The listing builds one solid part. Answer for the finished solid, in the listing's coordinates (mm). Round coordinates to 2 decimals unless told otherwise and drop trailing zeros. Write each loop counter-clockwise with the first axis right and the second up, starting at its lowest first coordinate (ties: lowest second). Pieces come first, ordered by that corner, then holes. Notation, with made-up numbers: (31, 47) - (77, 47) arc R26 ccw to (77, 71) - close; hole circle Ø4 at (69.5, -20.5). An arc over 180 degrees is marked (long way). Answer in a Markdown table with one row per item.
Autodesk Inventor part; units mm, degrees
ref_plane "YZ Plane" through (0, 0, 0) normal (1, 0, 0) x (0, 1, 0)
ref_plane "XZ Plane" through (0, 0, 0) normal (0, 1, 0) x (-1, 0, 0)
ref_plane "XY Plane" through (0, 0, 0) normal (0, 0, 1) x (1, 0, 0)
sketch "board" plane through (0, 0, 0) normal (0, 0, 1) x (1, 0, 0)
  line L0 (22.5, 10) -> (-22.5, 10)
  line L1 (-22.5, 10) -> (-22.5, -10)
  line L2 (-22.5, -10) -> (22.5, -10)
  line L3 (22.5, -10) -> (22.5, 10)
  line L4 (22.5, 10) -> (-22.5, -10) construction
  line L5 (-22.5, 10) -> (22.5, -10) construction
  circle A0 centre (-3.81, -8) radius 0.5
  circle A1 centre (-21.25, 8.75) radius 0.8
  circle A2 centre (21.25, 8.75) radius 0.8
  circle A3 centre (-21.25, -8.75) radius 0.8
  circle A4 centre (21.25, -8.75) radius 0.8
  circle A5 centre (-1.27, -8) radius 0.5
  circle A6 centre (1.27, -8) radius 0.5
  circle A7 centre (3.81, -8) radius 0.5
  circle A8 centre (-2.44, 7) radius 0.5
  circle A9 centre (2.44, 7) radius 0.5
  circle A10 centre (-13.1, 5.1) radius 0.75
  circle A11 centre (13.1, 5.1) radius 0.75
  circle A12 centre (-13.1, -5.1) radius 0.75
  circle A13 centre (13.1, -5.1) radius 0.75
  point P0 (0, 0)
  point P1 (0, 0)
  point P2 (13.2529, 5)
  dimension "d34" = 45
  dimension "d35" = 20
  dimension "d39" = 1
  dimension "d44" = 1.6
  dimension "d48" = 1.25
  dimension "d51" = 42.5
  dimension "d54" = 17.5
  dimension "d57" = 1.25
  dimension "d60" = 2.54
  dimension "d65" = 3.81
  dimension "d66" = 2
  dimension "d67" = 4.88
  dimension "d68" = 2.44
  dimension "d69" = 1
  dimension "d70" = 1
  dimension "d71" = 3
  dimension "d72" = 1.5
  dimension "d75" = 26.2
  dimension "d78" = 10.2
  dimension "d81" = 5.1
  dimension "d82" = 13.1
extrude "Extrusion2" add sketch "board" along normal blind 1.5
equation "\"d70\" = d69"
properties part number "Board"
(1) Section D-D (x = 21.25) is taken. Give the vertices of the cut face in (y, z), and give its area (3 significant figures).
Checked values:
| item | result |
|---|---|
| outline | (-10, 0) - (-9.55, 0) - (-9.55, 1.5) - (-10, 1.5) - close; (-7.95, 0) - (7.95, 0) - (7.95, 1.5) - (-7.95, 1.5) - close; (9.55, 0) - (10, 0) - (10, 1.5) - (9.55, 1.5) - close |
| area | 25.2 mm2 |
(2) Find the intervals of material crossed by line 1 (Y direction, x = -13.1, z = 0.65); line 2 (X direction, y = 5.5, z = 1.45); line 3 (Y direction, x = 13.5, z = 0.6), in increasing order.
Checked values:
| item | result |
|---|---|
| line 1 | y = -10 to -5.85, -4.35 to 4.35, 5.85 to 10 |
| line 2 | x = -22.5 to -13.73, -12.47 to 12.47, 13.73 to 22.5 |
| line 3 | y = -10 to -5.73, -4.47 to 4.47, 5.73 to 10 |
(3) Section B-B (y = 7) is taken. Give the vertices of the cut face in (x, z).
Checked values:
| item | result |
|---|---|
| outline | (-22.5, 0) - (-2.94, 0) - (-2.94, 1.5) - (-22.5, 1.5) - close; (-1.94, 0) - (1.94, 0) - (1.94, 1.5) - (-1.94, 1.5) - close; (2.94, 0) - (22.5, 0) - (22.5, 1.5) - (2.94, 1.5) - close |
(4) For a pull along Y with two mould halves and no side action, classify faces 1 (the flat face through (-22.5, 0, 1)), 2 (the cylindrical face through (-1.378, -7.512, 0.74)), 3 (the flat face through (0, -10, 1)) as pulls with the +Y half, pulls with the -Y half, needs draft (parallel to the pull), parting line crosses it, or undercut.
Checked values:
| item | result |
|---|---|
| face 1 | needs draft |
| face 2 | undercut |
| face 3 | pulls with the -Y half |
(5) Section A-A (x = -3.81) is taken. Give the vertices of the cut face in (y, z), and give its area (3 significant figures).
Checked values:
| item | result |
|---|---|
| outline | (-10, 0) - (-8.5, 0) - (-8.5, 1.5) - (-10, 1.5) - close; (-7.5, 0) - (10, 0) - (10, 1.5) - (-7.5, 1.5) - close |
| area | 28.5 mm2 |
(6) Section C-C (z = 0.25) is taken. State how many separate pieces and enclosed holes the cut face has, and give its area (3 significant figures).
Checked values:
| item | result |
|---|---|
| separate pieces | 1 |
| enclosed holes | 14 |
| area | 880 mm2 |
